```python
from build123d import *

# Parameters (mm, degrees)
F0_R     = 6.35
F1_DEPTH = 6.35


with BuildPart() as f1:
    # F0 (on Right) → F1 (new body)
    with BuildSketch(Plane.YZ):
        Polygon((0, 6.35), (0, 0), (254, 0), (254, 6.35), (247.65, 6.35), (247.65, 12.7), (254, 12.7), (254, 19.05), (247.65, 19.05), (247.65, 25.4), (254, 25.4), (254, 31.75), (247.65, 31.75), (247.65, 38.1), (254, 38.1), (254, 44.45), (247.65, 44.45), (247.65, 50.8), (254, 50.8), (254, 57.15), (127, 57.15), (0, 19.05), (0, 12.7), (6.35, 12.7), (6.35, 6.35), align=None)
        with Locations((127, 44.45)):
            Circle(F0_R, mode=Mode.SUBTRACT)
    extrude(amount=F1_DEPTH)


solid = f1.part
```
The listing builds one solid part. Answer for the finished solid, in the listing's coordinates (mm). A direction names the side the tool comes from. Round coordinates to 2 decimals unless told otherwise and drop trailing zeros. Loops run counter-clockwise (first coordinate to the right, second up) from the corner with the lowest first, then second, coordinate; pieces in that order, holes last.
1) For faces 4 (the face through (0, 153, 23)), 5 (the face through (3, 251, 44.45)), 6 (the face through (3, 6.35, 10)), determine the directions among +Z, -Z, +X, -X, +Y, -Y from which every point of the face is accessible in a straight line to the end or side of a thin tool.
Outcome:
face 4: +Z, -Z, -X, +Y, -Y
face 5: +X, -X, +Y
face 6: +X, -X, -Y
2) For a pull along Z with two mould halves and no side action, classify faces 1 (the face through (3, 0, 3)), 2 (the face through (3, 191, 57.15)), 3 (the face through (3, 251, 6.35)) as released by +Z, released by -Z, zero draft, split by the parting line, or undercut.
Outcome:
face 1: zero draft
face 2: released by +Z
face 3: undercut
3) A cutting plane is placed at D-D on z = 34.5. Determine the outline of the cut face in (x, y), plus the area to 3 significant figures.
Outcome:
outline: (0, 51.5) - (6.35, 51.5) - (6.35, 247.65) - (0, 247.65) - close
area: 1,250 mm2
4) A cutting plane is placed at B-B on z = 48. Determine the outline of the cut face in (x, y).
Outcome:
outline: (0, 96.5) - (6.35, 96.5) - (6.35, 121.74) - (0, 121.74) - close; (0, 132.26) - (6.35, 132.26) - (6.35, 247.65) - (0, 247.65) - close
5) Consider line 1 (Z direction, x = 5.25, y = 127); line 2 (Z direction, x = 6, y = 24); line 3 (Z direction, x = 5.25, y = 62). Determine where each line is inside the solid, lowest interval first.
Outcome:
line 1: z = 0 to 38.1, 50.8 to 57.15
line 2: z = 0 to 26.25
line 3: z = 0 to 37.65
6) Given P1, Ø1.9, axis at x = 3, z = 8.5, coming from the -Y side; P2, Ø3, axis at x = 4, y = 3, coming from the -Z side; P3, Ø2, axis at x = 1, y = 46, coming from the +Z side; P4, Ø3, axis at x = 4, z = 9.5, coming from the +Y side, each flat-ended and moving along its own axis, determine where each tip first touches the part or whether it passes through.
Outcome:
P1: stops at y = 6.35
P2: stops at z = 0
P3: stops at z = 33.15
P4: stops at y = 247.65
7) A cutting plane is placed at C-C on y = 63.5. Determine the outline of the cut face in (x, z).
Outcome:
outline: (0, 0) - (6.35, 0) - (6.35, 38.1) - (0, 38.1) - close
8) A cutting plane is placed at A-A on x = 3. Determine the outline of the cut face in (y, z).
Outcome:
outline: (0, 0) - (254, 0) - (254, 6.35) - (247.65, 6.35) - (247.65, 12.7) - (254, 12.7) - (254, 19.05) - (247.65, 19.05) - (247.65, 25.4) - (254, 25.4) - (254, 31.75) - (247.65, 31.75) - (247.65, 38.1) - (254, 38.1) - (254, 44.45) - (247.65, 44.45) - (247.65, 50.8) - (254, 50.8) - (254, 57.15) - (127, 57.15) - (0, 19.05) - (0, 12.7) - (6.35, 12.7) - (6.35, 6.35) - (0, 6.35) - close; hole circle Ø12.7 at (127, 44.45)
